Build history of the part. All positions in model axes, mm. A direction names the side the tool comes from. Give positions to 0.01 mm unless a question says otherwise; leave off trailing zeros. Loops run counter-clockwise (first coordinate to the right, second up) from the corner with the lowest first, then second, coordinate; pieces in that order, holes last. Notation, with made-up numbers: (53, 73.5) -> (111, 73.5) arc R27 cw to (111, 102.5) -> close; hole circle Ø2 at (-6, 17.25). An arc over 180 degrees is marked (long way). Answer in a Markdown table with one row per item. Add a question column.
from build123d import *

# Parameters (mm, degrees)
SKETCH2_W           = 112
SKETCH2_H           = 73
BOSS_EXTRUDE1_DEPTH = 50
SHELL3_T            = -3
SKETCH5_R           = 4
BOSS_EXTRUDE2_DEPTH = 47.5
CUT_EXTRUDE1_REACH  = 75
SKETCH3_W           = 72
SKETCH3_H           = 26
SKETCH6_R           = 1.47
CUT_EXTRUDE2_DEPTH  = 10
FILLET1_R           = 4
CUT_EXTRUDE3_REACH  = 75
SKETCH7_R           = 1.35
CUT_EXTRUDE4_REACH  = 75
SKETCH8_R           = 5
CUT_EXTRUDE5_REACH  = 114
SKETCH9_R           = 5


with BuildPart() as part:
    # Sketch2 → Boss-Extrude1 (new body)
    with BuildSketch(Plane(origin=(0, 0, 0), x_dir=(1, 0, 0), z_dir=(0, 1, 0))):
        Rectangle(SKETCH2_W, SKETCH2_H)
    extrude(amount=BOSS_EXTRUDE1_DEPTH)

    # Shell3
    shell3_openings = [part.faces().sort_by_distance(p)[0] for p in [
        (0, 50, 0),
    ]]
    offset(amount=SHELL3_T, openings=shell3_openings, kind=Kind.INTERSECTION)

    # Sketch5 → Boss-Extrude2 (add)
    with BuildSketch(Plane(origin=(0, 2.5, 0), x_dir=(1, 0, 0), z_dir=(0, 1, 0))):
        with Locations((-51, 31.5)):
            Circle(SKETCH5_R)
        with Locations((-51, -31.5)):
            Circle(SKETCH5_R)
        with Locations((51, 31.5)):
            Circle(SKETCH5_R)
        with Locations((51, -31.5)):
            Circle(SKETCH5_R)
    extrude(amount=BOSS_EXTRUDE2_DEPTH)

    # Sketch3 → Cut-Extrude1 (cut, up to next)
    with BuildSketch(Plane.XY.offset(36.5), mode=Mode.PRIVATE) as cut_extrude1_sk1:
        with Locations((0, 25)):
            Rectangle(SKETCH3_W, SKETCH3_H)
    cut_extrude1_tool1 = extrude(cut_extrude1_sk1.sketch, amount=-CUT_EXTRUDE1_REACH, mode=Mode.PRIVATE) & part.part
    add(cut_extrude1_tool1.solids().sort_by_distance((0, 25, 36.5))[0], mode=Mode.SUBTRACT)

    # Sketch6 → Cut-Extrude2 (cut)
    with BuildSketch(Plane(origin=(0, 50, 0), x_dir=(1, 0, 0), z_dir=(0, 1, 0))):
        with Locations((51, 31.5)):
            Circle(SKETCH6_R)
        with Locations((51, -31.5)):
            Circle(SKETCH6_R)
        with Locations((-51, -31.5)):
            Circle(SKETCH6_R)
        with Locations((-51, 31.5)):
            Circle(SKETCH6_R)
    extrude(amount=-CUT_EXTRUDE2_DEPTH, mode=Mode.SUBTRACT)

    # Fillet1
    fillet1_edges = [part.edges().sort_by_distance(p)[0] for p in [
        (56, 25, 36.5),
        (-56, 25, 36.5),
        (-56, 25, -36.5),
        (56, 25, -36.5),
    ]]
    fillet(fillet1_edges, radius=FILLET1_R)

    # Sketch7 → Cut-Extrude3 (cut, up to next)
    with BuildSketch(Plane.XY.offset(36.5), mode=Mode.PRIVATE) as cut_extrude3_sk1:
        with Locations((-37.26, 40.74)):
            Circle(SKETCH7_R)
    cut_extrude3_tool1 = extrude(cut_extrude3_sk1.sketch, amount=-CUT_EXTRUDE3_REACH, mode=Mode.PRIVATE) & part.part
    add(cut_extrude3_tool1.solids().sort_by_distance((-37.26, 40.74, 36.5))[0], mode=Mode.SUBTRACT)
    # Sketch7 → Cut-Extrude3 (cut, up to next)
    with BuildSketch(Plane.XY.offset(36.5), mode=Mode.PRIVATE) as cut_extrude3_sk2:
        with Locations((-37.26, 9.26)):
            Circle(SKETCH7_R)
    cut_extrude3_tool2 = extrude(cut_extrude3_sk2.sketch, amount=-CUT_EXTRUDE3_REACH, mode=Mode.PRIVATE) & part.part
    add(cut_extrude3_tool2.solids().sort_by_distance((-37.26, 9.26, 36.5))[0], mode=Mode.SUBTRACT)
    # Sketch7 → Cut-Extrude3 (cut, up to next)
    with BuildSketch(Plane.XY.offset(36.5), mode=Mode.PRIVATE) as cut_extrude3_sk3:
        with Locations((37.26, 40.74)):
            Circle(SKETCH7_R)
    cut_extrude3_tool3 = extrude(cut_extrude3_sk3.sketch, amount=-CUT_EXTRUDE3_REACH, mode=Mode.PRIVATE) & part.part
    add(cut_extrude3_tool3.solids().sort_by_distance((37.26, 40.74, 36.5))[0], mode=Mode.SUBTRACT)
    # Sketch7 → Cut-Extrude3 (cut, up to next)
    with BuildSketch(Plane.XY.offset(36.5), mode=Mode.PRIVATE) as cut_extrude3_sk4:
        with Locations((37.26, 9.26)):
            Circle(SKETCH7_R)
    cut_extrude3_tool4 = extrude(cut_extrude3_sk4.sketch, amount=-CUT_EXTRUDE3_REACH, mode=Mode.PRIVATE) & part.part
    add(cut_extrude3_tool4.solids().sort_by_distance((37.26, 9.26, 36.5))[0], mode=Mode.SUBTRACT)

    # Sketch8 → Cut-Extrude4 (cut, up to next)
    with BuildSketch(Plane(origin=(0, 0, -36.5), x_dir=(-1, 0, 0), z_dir=(0, 0, -1)), mode=Mode.PRIVATE) as cut_extrude4_sk1:
        with Locations((0, 25)):
            Circle(SKETCH8_R)
    cut_extrude4_tool1 = extrude(cut_extrude4_sk1.sketch, amount=-CUT_EXTRUDE4_REACH, mode=Mode.PRIVATE) & part.part
    add(cut_extrude4_tool1.solids().sort_by_distance((0, 25, -36.5))[0], mode=Mode.SUBTRACT)

    # Sketch9 → Cut-Extrude5 (cut, up to next)
    with BuildSketch(Plane.ZY.offset(56), mode=Mode.PRIVATE) as cut_extrude5_sk1:
        with Locations((0, 25)):
            Circle(SKETCH9_R)
    cut_extrude5_tool1 = extrude(cut_extrude5_sk1.sketch, amount=-CUT_EXTRUDE5_REACH, mode=Mode.PRIVATE) & part.part
    add(cut_extrude5_tool1.solids().sort_by_distance((-56, 25, 0))[0], mode=Mode.SUBTRACT)


solid = part.part
(1) Two-plate mould, pull along Y, no slides. Class faces 1 (the flat face through (-1, 31, -33.5)), 2 (the flat face through (-1, 38, 35)), 3 (the flat face through (-51, 40, 31)): released by +Y, released by -Y, zero draft, split by the parting line, or undercut.
(2) Flat gauge pins, fed straight in: pin 1 Ø2.5 at (x, z) = (51, -31.5) entering from +Y; pin 2 Ø1 at (x, z) = (-35, 0.5) entering from +Y; pin 3 Ø10 at (x, y) = (10, 22.5) entering from +Z. Where does each tip first touch, or does it go through?
(3) Saw through at D-D, the plane x = -37.26. List the corners of the cut face in (y, z).
(4) Wall check: line 1 along Z through (x, y) = (-51, 46.5); line 2 along X through (y, z) = (10, 22.5); line 3 along Z through (x, y) = (29.5, 6.5). Give the ranges that are in metal, low to high. Write a range as from..to.
(5) Saw through at A-A, the plane x = 22.5. List the corners of the cut face in (y, z), then the cut area to 3 significant figures.
(6) Saw through at B-B, the plane y = 44. List the corners of the cut face in (x, z), then the cut area to 3 significant figures.
(7) 3-axis set-ups, long thin cutter, end or side, ignore diameter. For faces 4 (the cylindrical face through (36.19, 39.92, 35.02)), 5 (the flat face through (56, 25, 0)), 6 (the flat face through (53, 26, 0)): which of +Z, -Z, +X, -X, +Y, -Y reach the whole face in a straight line?
(8) Saw through at C-C, the plane z = 1. List the corners of the cut face in (x, y), then the cut area to 3 significant figures.
Worked answers:
| question | item | result |
|---|---|---|
| 1 | face 1 | zero draft |
| 1 | face 2 | undercut |
| 1 | face 3 | released by +Y |
| 2 | pin 1 | y = 40 |
| 2 | pin 2 | y = 3 |
| 2 | pin 3 | z = -33.5 |
| 3 | outline | (0, -36.5) -> (50, -36.5) -> (50, -33.5) -> (3, -33.5) -> (3, 33.5) -> (7.91, 33.5) -> (7.91, 36.5) -> (0, 36.5) -> close; (10.61, 33.5) -> (39.39, 33.5) -> (39.39, 36.5) -> (10.61, 36.5) -> close; (42.09, 33.5) -> (50, 33.5) -> (50, 36.5) -> (42.09, 36.5) -> close |
| 4 | line 1 | -36.5..-32.97, -30.03..-27.5, 27.5..30.03, 32.97..36.5 |
| 4 | line 2 | -56..-53, 53..56 |
| 4 | line 3 | -36.5..-33.5, 33.5..36.5 |
| 5 | outline | (0, -36.5) -> (50, -36.5) -> (50, -33.5) -> (3, -33.5) -> (3, 33.5) -> (12, 33.5) -> (12, 36.5) -> (0, 36.5) -> close; (38, 33.5) -> (50, 33.5) -> (50, 36.5) -> (38, 36.5) -> close |
| 5 | area | 423 mm^2 |
| 6 | outline | (-56, -32.5) arc R4 ccw to (-52, -36.5) -> (52, -36.5) arc R4 ccw to (56, -32.5) -> (56, 32.5) arc R4 ccw to (52, 36.5) -> (-52, 36.5) arc R4 ccw to (-56, 32.5) -> close; hole (-53, -28.04) arc R4 cw to (-47.54, -33.5) -> (47.54, -33.5) arc R4 cw to (53, -28.04) -> (53, 28.04) arc R4 cw to (47.54, 33.5) -> (-47.54, 33.5) arc R4 cw to (-53, 28.04) -> close; hole circle Ø2.94 at (-51, -31.5); hole circle Ø2.94 at (-51, 31.5); hole circle Ø2.94 at (51, -31.5); hole circle Ø2.94 at (51, 31.5) |
| 6 | area | 1,160 mm^2 |
| 7 | face 4 | +Z |
| 7 | face 5 | +Z, -Z, +X, +Y, -Y |
| 7 | face 6 | +Y |
| 8 | outline | (-56, 0) -> (56, 0) -> (56, 50) -> (53, 50) -> (53, 3) -> (-53, 3) -> (-53, 20.1) -> (-56, 20.1) -> close; (-56, 29.9) -> (-53, 29.9) -> (-53, 50) -> (-56, 50) -> close |
| 8 | area | 589 mm^2 |
